Work out the finished part from the listing and answer in its coordinate system (mm). A direction names the side the tool comes from. Give positions to 0.01 mm unless a question says otherwise; leave off trailing zeros. Loops run counter-clockwise (first coordinate to the right, second up) from the corner with the lowest first, then second, coordinate; pieces in that order, holes last. Notation, with made-up numbers: (2.25, 85.25) - (28.25, 85.25) arc R13 cw to (28.25, 103.25) - close; hole circle Ø4 at (61, -1.5). An arc over 180 degrees is marked (long way). Use CSV: the item, a comma, the result in double quotes.
from build123d import *

# Parameters (mm, degrees)
SKETCH1_R           = 19.05
SKETCH1_R_2         = 13.9954
BOSS_EXTRUDE1_DEPTH = 63.5
SKETCH2_R           = 19.05
BOSS_EXTRUDE2_DEPTH = 12.7
SKETCH3_R           = 12.7
BOSS_EXTRUDE3_DEPTH = 127
FILLET1_R           = 0.508
CHAMFER1_SIZE       = 1.27
CUT_EXTRUDE1_DEPTH  = 76.2
FILLET2_R           = 3.175
BOSS_EXTRUDE4_DEPTH = 76.2
BOSS_EXTRUDE5_START = 63.5
SKETCH6_R           = 13.9954
BOSS_EXTRUDE5_DEPTH = 63.5
SKETCH7_R           = 25.219402827
SKETCH7_R_2         = 12.7
CUT_EXTRUDE2_DEPTH  = 63.5
SKETCH8_R           = 14.2875
CUT_EXTRUDE3_DEPTH  = 19.05
SKETCH9_W           = 6.35
SKETCH9_H           = 41.275
CUT_EXTRUDE4_DEPTH  = 25.4
FILLET3_R           = 3.175
SKETCH10_R          = 33.957183176
CUT_EXTRUDE5_DEPTH  = 44.45
SKETCH11_R          = 19.05
SKETCH11_R_2        = 14.986
BOSS_EXTRUDE6_DEPTH = 20.2184
SKETCH12_R          = 18.486840379
CUT_EXTRUDE6_DEPTH  = 25.4
SKETCH13_R          = 16.938517856
SKETCH13_R_2        = 11.938
CUT_EXTRUDE7_DEPTH  = 1.1684
CHAMFER3_SIZE       = 0.508


with BuildPart() as part:
    # Sketch1 → Boss-Extrude1 (new body)
    with BuildSketch(Plane.XY):
        Circle(SKETCH1_R)
        Circle(SKETCH1_R_2, mode=Mode.SUBTRACT)
    extrude(amount=BOSS_EXTRUDE1_DEPTH)

    # Sketch2 → Boss-Extrude2 (add)
    with BuildSketch(Plane.XY.offset(63.5)):
        Circle(SKETCH2_R)
    extrude(amount=BOSS_EXTRUDE2_DEPTH)

    # Sketch3 → Boss-Extrude3 (add)
    with BuildSketch(Plane.XY.offset(76.2)):
        Circle(SKETCH3_R)
    extrude(amount=BOSS_EXTRUDE3_DEPTH)

    # Fillet1
    fillet1_edges = [part.edges().sort_by_distance(p)[0] for p in [
        (-12.7, 0, 76.2),
    ]]
    fillet(fillet1_edges, radius=FILLET1_R)

    # Chamfer1
    chamfer1_edges = [part.edges().sort_by_distance(p)[0] for p in [
        (-12.7, 0, 203.2),
    ]]
    chamfer(chamfer1_edges, length=CHAMFER1_SIZE)

    # Sketch4 → Cut-Extrude1 (cut)
    with BuildSketch(Plane.XY.offset(78.74)):
        with BuildLine():
            Line((-3.175, 9.525), (3.175, 9.525))
            Line((3.175, 9.525), (3.175, 12.296722124))
            ThreePointArc((3.175, 12.296722124), (0, 12.7), (-3.175, 12.296722124))
            Line((-3.175, 12.296722124), (-3.175, 9.525))
        make_face()
    extrude(amount=CUT_EXTRUDE1_DEPTH, mode=Mode.SUBTRACT)

    # Fillet2
    fillet2_edges = [part.edges().sort_by_distance(p)[0] for p in [
        (3.175, 10.910861062, 154.94),
        (-3.175, 10.910861062, 154.94),
        (3.175, 10.910861062, 78.74),
        (-3.175, 10.910861062, 78.74),
    ]]
    fillet(fillet2_edges, radius=FILLET2_R - 0.0001)  # a hair under: the kernel refuses the full size

    # Sketch5 → Boss-Extrude4 (add)
    with BuildSketch(Plane(origin=(0, 0, 0), x_dir=(-1, 0, 0), z_dir=(0, 0, -1))):
        with BuildLine():
            Line((-4.6e-08, 19.05), (-11.4476253, 19.05))
            ThreePointArc((-11.4476253, 19.05), (-22.225, 0), (-11.4476253, -19.05))
            Line((-11.4476253, -19.05), (1.9e-08, -19.05))
            ThreePointArc((1.9e-08, -19.05), (-19.05, -3.2e-08), (-4.6e-08, 19.05))
        make_face()
        with BuildLine():
            Line((11.4476253, 19.05), (-4.6e-08, 19.05))
            ThreePointArc((-4.6e-08, 19.05), (13.470384166, 13.470384198), (19.05, 0))
            ThreePointArc((19.05, 0), (13.470384188, -13.470384175), (1.9e-08, -19.05))
            Line((1.9e-08, -19.05), (11.4476253, -19.05))
            ThreePointArc((11.4476253, -19.05), (19.343915029, -10.943654616), (22.225, 0))
            ThreePointArc((22.225, 0), (19.343915029, 10.943654616), (11.4476253, 19.05))
        make_face()
    extrude(amount=-BOSS_EXTRUDE4_DEPTH)

    # Sketch6 → Boss-Extrude5 (add)
    with BuildSketch(Plane(origin=(0, 0, 63.5), x_dir=(-1, 0, 0), z_dir=(0, 0, -1)).offset(BOSS_EXTRUDE5_START)):
        Circle(SKETCH6_R)
    extrude(amount=-BOSS_EXTRUDE5_DEPTH)

    # Sketch7 → Cut-Extrude2 (cut)
    with BuildSketch(Plane(origin=(0, 0, 0), x_dir=(-1, 0, 0), z_dir=(0, 0, -1))):
        Circle(SKETCH7_R)
        with Locations(Location((0, 0, 0), (0, 0, 180))):
            Circle(SKETCH7_R_2, mode=Mode.SUBTRACT)
    extrude(amount=-CUT_EXTRUDE2_DEPTH, mode=Mode.SUBTRACT)

    # Sketch8 → Cut-Extrude3 (cut)
    with BuildSketch(Plane(origin=(0, 0, 0), x_dir=(-1, 0, 0), z_dir=(0, 0, -1))):
        Circle(SKETCH8_R)
    extrude(amount=-CUT_EXTRUDE3_DEPTH, mode=Mode.SUBTRACT)

    # Sketch9 → Cut-Extrude4 (cut)
    with BuildSketch(Plane(origin=(0, 9.525, 0), x_dir=(1, 0, 0), z_dir=(0, 1, 0))):
        with Locations((0, -39.6875)):
            Rectangle(SKETCH9_W, SKETCH9_H)
    extrude(amount=CUT_EXTRUDE4_DEPTH, mode=Mode.SUBTRACT)

    # Fillet3
    fillet3_edges = [part.edges().sort_by_distance(p)[0] for p in [
        (-3.175, 10.910861062, 60.325),
        (3.175, 10.910861062, 60.325),
    ]]
    fillet(fillet3_edges, radius=FILLET3_R - 0.0001)  # a hair under: the kernel refuses the full size

    # Sketch10 → Cut-Extrude5 (cut)
    with BuildSketch(Plane(origin=(0, 0, 19.05), x_dir=(-1, 0, 0), z_dir=(0, 0, -1))):
        Circle(SKETCH10_R)
    extrude(amount=-CUT_EXTRUDE5_DEPTH, mode=Mode.SUBTRACT)

    # Sketch11 → Boss-Extrude6 (add)
    with BuildSketch(Plane(origin=(0, 0, 63.5), x_dir=(-1, 0, 0), z_dir=(0, 0, -1))):
        with Locations(Location((0, 0, 0), (0, 0, 270))):
            Circle(SKETCH11_R)
        Circle(SKETCH11_R_2, mode=Mode.SUBTRACT)
    extrude(amount=BOSS_EXTRUDE6_DEPTH)

    # Sketch12 → Cut-Extrude6 (cut)
    with BuildSketch(Plane.XY.offset(203.2)):
        Circle(SKETCH12_R)
    extrude(amount=-CUT_EXTRUDE6_DEPTH, mode=Mode.SUBTRACT)

    # Sketch13 → Cut-Extrude7 (cut)
    with BuildSketch(Plane.XY.offset(175.006)):
        Circle(SKETCH13_R)
        Circle(SKETCH13_R_2, mode=Mode.SUBTRACT)
    extrude(amount=CUT_EXTRUDE7_DEPTH, mode=Mode.SUBTRACT)

    # Chamfer3
    chamfer3_edges = [part.edges().sort_by_distance(p)[0] for p in [
        (-12.7, 0, 177.8),
    ]]
    chamfer(chamfer3_edges, length=CHAMFER3_SIZE)


solid = part.part
Item 1: For faces 5 (the cylindrical face through (-2.22, 11.09, 154.035)), 6 (the flat face through (19.4, 1.5, 63.5)), 7 (the flat face through (-19.3, 0.1, 63.5)), determine the directions among +Z, -Z, +X, -X, +Y, -Y from which every point of the face is accessible in a straight line to the end or side of a thin tool.
Determined:
face 5,"+Y"
face 6,"-Z, +X"
face 7,"-Z, -X"
Item 2: The mould has two halves that part along X. Classify faces 1 (the flat face through (11.2, -4.6, 175.006)), 2 (the cylindrical face through (-2.27, 11.09, 79.695)), 3 (the flat face through (0, 9.525, 116)), 4 (the cylindrical face through (22.223, 0.32, 69.761)): pulls with the +X half, pulls with the -X half, needs draft (parallel to the pull), parting line crosses it, or undercut.
Determined:
face 1,"needs draft"
face 2,"undercut"
face 3,"undercut"
face 4,"pulls with the +X half"
Item 3: Given P1, Ø4, axis at x = 15.5, z = 72, coming from the -Y side; P2, Ø2, axis at x = -5.5, z = 128.5, coming from the +Y side; P3, Ø4, axis at x = -11, y = -1, coming from the -Z side, each flat-ended and moving along its own axis, determine where each tip first touches the part or whether it passes through.
Determined:
P1,"stops at y = -17.66"
P2,"stops at y = 11.88"
P3,"stops at z = 63.5"
Item 4: A cutting plane is placed at A-A on z = 112. Determine the outline of the cut face in (x, y) (3 decimals), and give its area (3 significant figures).
Determined:
outline,"(-3.175, 9.525) - (-3.175, 12.297) arc R12.7 ccw (long way) to (3.175, 12.297) - (3.175, 9.525) - close"
area,"487 mm²"
Item 5: Find the intervals of material crossed by line 1 (Z direction, x = 5, y = -5); line 2 (Z direction, x = 9, y = 16.5); line 3 (X direction, y = 3.5, z = 62), in increasing order.
Determined:
line 1,"z = 63.5 to 177.8"
line 2,"z = 43.28 to 76.2"
line 3,"x = -18.73 to -14.57, 14.57 to 18.73"
